Design review of the part shown in the three views and the two pictorial views. Dimensions are in mm from the part's minimum x, y and z. Round coordinates to 2 decimals unless told otherwise and drop trailing zeros. Order: outer loops, then holes, each group sorted by start corner. A loop starts at its lowest first (then second) coordinate and runs counter-clockwise, first axis right, second up. Notation, with made-up numbers: (8.5, 19) -> (37.5, 19) arc R30 ccw to (37.5, 53) -> close; hole circle Ø3 at (31.25, 46). An arc over 180 degrees is marked (long way). Put each result on its own line as item: value. Start each with the question number.
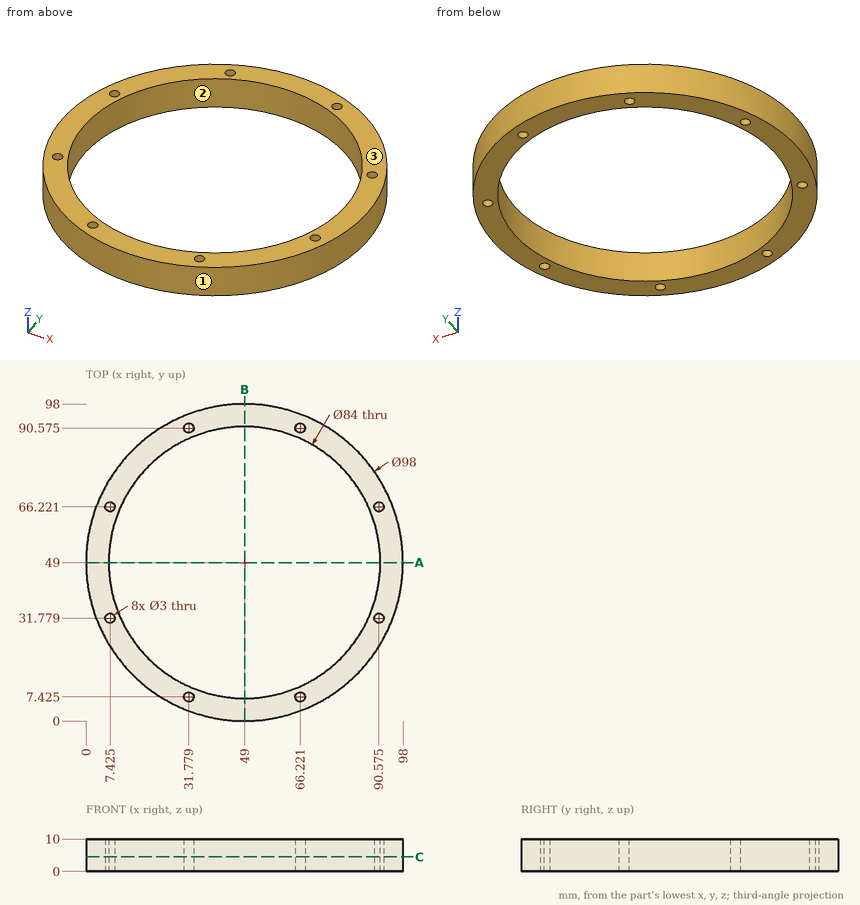
Q1. Draft analysis for pull direction Y (two halves, no side actions). For the marked faces 1, 2 and 3, state which applies: +Y half, -Y half, draft (parallel to the pull), parting line (faces both ways), or undercut.
Q2. Take a section at A-A on y = 49. Give the boundary of the cut face in (x, z).
Q3. Take a section at C-C on z = 4.5. State how many separate pieces and enclosed holes the cut face has.
Q4. Wall thickness on probe 1 along Y at (x, z) = (49.5, 6); probe 2 along X at (y, z) = (17, 4.75) (1 decimal); probe 3 along Y at (x, z) = (68.5, 8): over which ranges is each line inside the solid? List them lowest first. Write a range as [from, to].
Q5. Clearance check with flat-ended pins moving along their axes: pin 1 Ø1.5 at (y, z) = (47.5, 7.5) entering from +X; pin 2 Ø5 at (x, z) = (56, 4.5) entering from +Y; pin 3 Ø4 at (y, z) = (43.5, 6) entering from -X (1 decimal). State where each tip first meets the part, or that it passes through.
Calculated:
1. face 1: parting line
1. face 2: undercut
1. face 3: draft
2. outline: (0, 0) -> (7, 0) -> (7, 10) -> (0, 10) -> close; (91, 0) -> (98, 0) -> (98, 10) -> (91, 10) -> close
3. separate pieces: 1
3. enclosed holes: 9
4. probe 1: y = [0, 7], [91, 98]
4. probe 2: x = [11.9, 21.8], [76.2, 86.1]
4. probe 3: y = [4.05, 11.8], [86.2, 93.95]
5. pin 1: stops at x = 97.99
5. pin 2: stops at y = 97.79
5. pin 3: stops at x = 0.1
